Verification items for the finished model (mm, model axes). Face numbers are marked on the shaded views. A direction names the side the tool comes from. Give positions to 0.01 mm unless a question says otherwise; leave off trailing zeros. Loops run counter-clockwise (first coordinate to the right, second up) from the corner with the lowest first, then second, coordinate; pieces in that order, holes last. Notation, with made-up numbers: (-32, 2) - (-25, 2) arc R35 cw to (-25, 37) - close; hole circle Ø9 at (9.25, -24). An arc over 180 degrees is marked (long way). Answer in a Markdown table with one row per item.
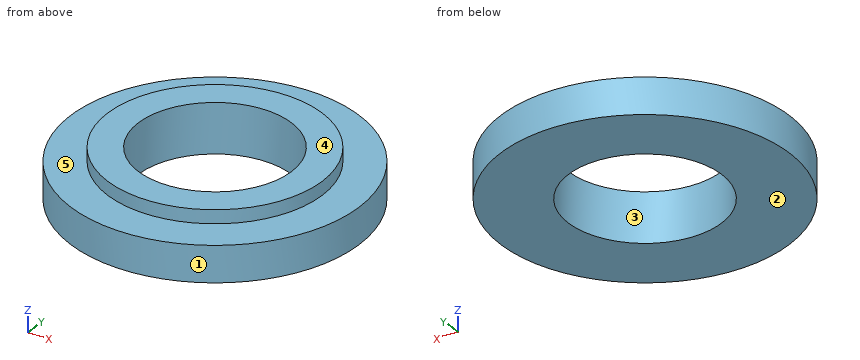
```python
from build123d import *

# Parameters (mm, degrees)
SKETCH001_R      = 8
SKETCH001_R_2    = 4.25
EXTRUDE001_DEPTH = 2
SKETCH_R         = 5.95
SKETCH_R_2       = 4.25
EXTRUDE_DEPTH    = 2.75


with BuildPart() as extrude001:
    # Sketch001 → Extrude001 (new body)
    with BuildSketch(Plane.XY):
        Circle(SKETCH001_R)
        Circle(SKETCH001_R_2, mode=Mode.SUBTRACT)
    extrude(amount=EXTRUDE001_DEPTH)


with BuildPart() as fusion:
    # Sketch → Extrude (new body)
    with BuildSketch(Plane.XY):
        Circle(SKETCH_R)
        Circle(SKETCH_R_2, mode=Mode.SUBTRACT)
    extrude(amount=EXTRUDE_DEPTH)

    # Fusion: union Extrude001
    add(extrude001.part)


solid = fusion.part
```
Q1. Tool access check on the marked faces 4 and 5. Record the directions out of +Z, -Z, +X, -X, +Y, -Y that give a thin tool (end or side, any length) a straight path to the whole face; none if there is none.
Completed:
| item | result |
|---|---|
| face 4 | +Z, +X, -X, +Y, -Y |
| face 5 | +Z |
Q2. Go/stop test with a flat-tipped pin: P1, Ø8, axis at x = -3, y = -0.5, coming from the +Z side. Record where the tip stops, or that it passes through.
Completed:
| item | result |
|---|---|
| P1 | z = 2.75 |
Q3. Draft check along X on the marked faces 1, 2 and 3. Enter one of: +X half, -X half, draft (parallel to the pull), parting line (faces both ways), or undercut.
Completed:
| item | result |
|---|---|
| face 1 | parting line |
| face 2 | draft |
| face 3 | undercut |
Q4. Sectioned sample at A-A (y = 0). Record the cut outline in (x, z), and give its area (4 significant figures).
Completed:
| item | result |
|---|---|
| outline | (-8, 0) - (-4.25, 0) - (-4.25, 2.75) - (-5.95, 2.75) - (-5.95, 2) - (-8, 2) - close; (4.25, 0) - (8, 0) - (8, 2) - (5.95, 2) - (5.95, 2.75) - (4.25, 2.75) - close |
| area | 17.55 mm^2 |
Q5. Sectioned sample at D-D (y = 5.5). Record the cut outline in (x, z).
Completed:
| item | result |
|---|---|
| outline | (-5.81, 0) - (5.81, 0) - (5.81, 2) - (2.27, 2) - (2.27, 2.75) - (-2.27, 2.75) - (-2.27, 2) - (-5.81, 2) - close |
Q6. Thickness scan on line 1 (Y direction, x = 0, z = 0.95); line 2 (Z direction, x = -5.5, y = 3); line 3 (X direction, y = -2, z = 2.6). Record the ranges inside material, lowest first.
Completed:
| item | result |
|---|---|
| line 1 | -8 to -4.25, 4.25 to 8 |
| line 2 | 0 to 2 |
| line 3 | -5.6 to -3.75, 3.75 to 5.6 |
Q7. Sectioned sample at C-C (z = 1.75). Record the cut outline in (x, y).
Completed:
| item | result |
|---|---|
| outline | circle Ø16 at (0, 0); hole circle Ø8.5 at (0, 0) |
